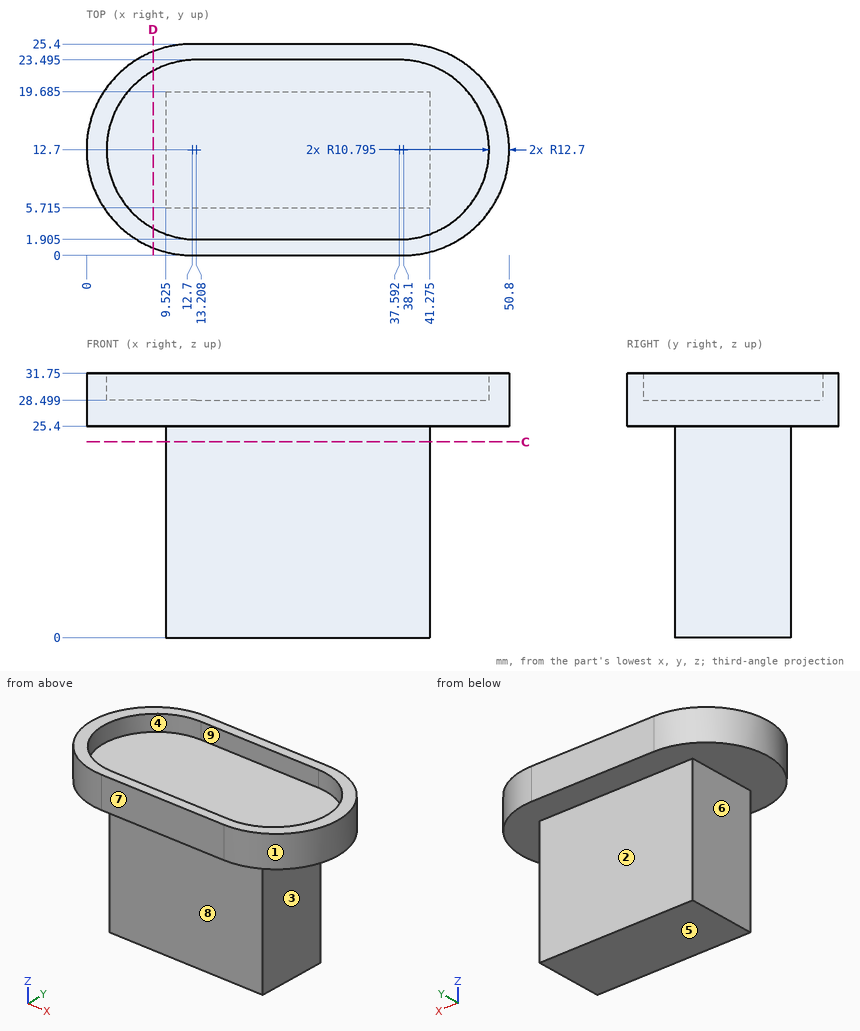
Can you work these out from the drawing? Everything is in mm from the part's minimum corner. A direction names the side the tool comes from. Round coordinates to 2 decimals unless told otherwise and drop trailing zeros. Write each loop counter-clockwise with the first axis right and the second up, starting at its lowest first coordinate (ties: lowest second). Pieces come first, ordered by that corner, then holes.
1. Suppose I cut it at C-C (z = 23.5). List the corners of the cut face in (x, y) for me (3 decimals), and give its area (3 significant figures).
2. If we mould it in two halves opening along Y, with no side actions, what happens to the marked faces 1, 2, 3 and 4? For each: released by +Y, released by -Y, zero draft, split by the parting line, or undercut.
3. Suppose I cut it at D-D (x = 8). List the corners of the cut face in (y, z) for me.
4. Will these pins go through, and if not, where does the flat tip stop? pin 1 Ø1.5 at (x, y) = (13, 18.5) entering from +Z; pin 2 Ø5 at (y, z) = (6.5, 28) entering from -X; pin 3 Ø8 at (y, z) = (3, 17) entering from -X (3 decimals).
5. For the marked faces 5, 6, 7, 8 and 9, which set-ups out of +Z, -Z, +X, -X, +Y, -Y let a thin tool reach every point of the face, with its end or its side?
6. I need wall thicknesses on L1, parallel to X at y = 12.25, z = 29; L2, parallel to Z at x = 9, y = 17; L3, parallel to Y at x = 13.5, z = 24 (3 decimals). Which ranges of each line are inside material? Lowest first, please.
Answer sheet:
1. outline: (9.525, 5.715) - (41.275, 5.715) - (41.275, 19.685) - (9.525, 19.685) - close
1. area: 444 mm2
2. face 1: split by the parting line
2. face 2: released by +Y
2. face 3: zero draft
2. face 4: undercut
3. outline: (0.9, 25.4) - (24.5, 25.4) - (24.5, 31.75) - (22.16, 31.75) - (22.16, 28.5) - (3.24, 28.5) - (3.24, 31.75) - (0.9, 31.75) - close
4. pin 1: stops at z = 28.5
4. pin 2: stops at x = 0.55
4. pin 3: stops at x = 9.525
5. face 5: -Z, +X, -X, +Y, -Y
5. face 6: -Z, -X, +Y, -Y
5. face 7: +Z, -Z, +X, -X, -Y
5. face 8: -Z, +X, -X, -Y
5. face 9: +Z
6. L1: x = 0.01 to 2.42, 48.38 to 50.79
6. L2: z = 25.4 to 28.5
6. L3: y = 5.715 to 19.685
